Input: dimensioned drawing with shaded views. Units: mm. Origin: part minimum x, y, z. A direction names the side the tool comes from. Give positions to 0.01 mm unless a question says otherwise; leave off trailing zeros. Order: outer loops, then holes, each group sorted by start corner. A loop starts at its lowest first (then second) coordinate and runs counter-clockwise, first axis right, second up. Notation, with made-up numbers: (-30.5, 3.25) - (22.5, 3.25) arc R14 ccw to (22.5, 12.25) - close; hole circle Ø8 at (79.5, 72.5). An arc over 180 degrees is marked (long way). Use a Markdown table: item, result.
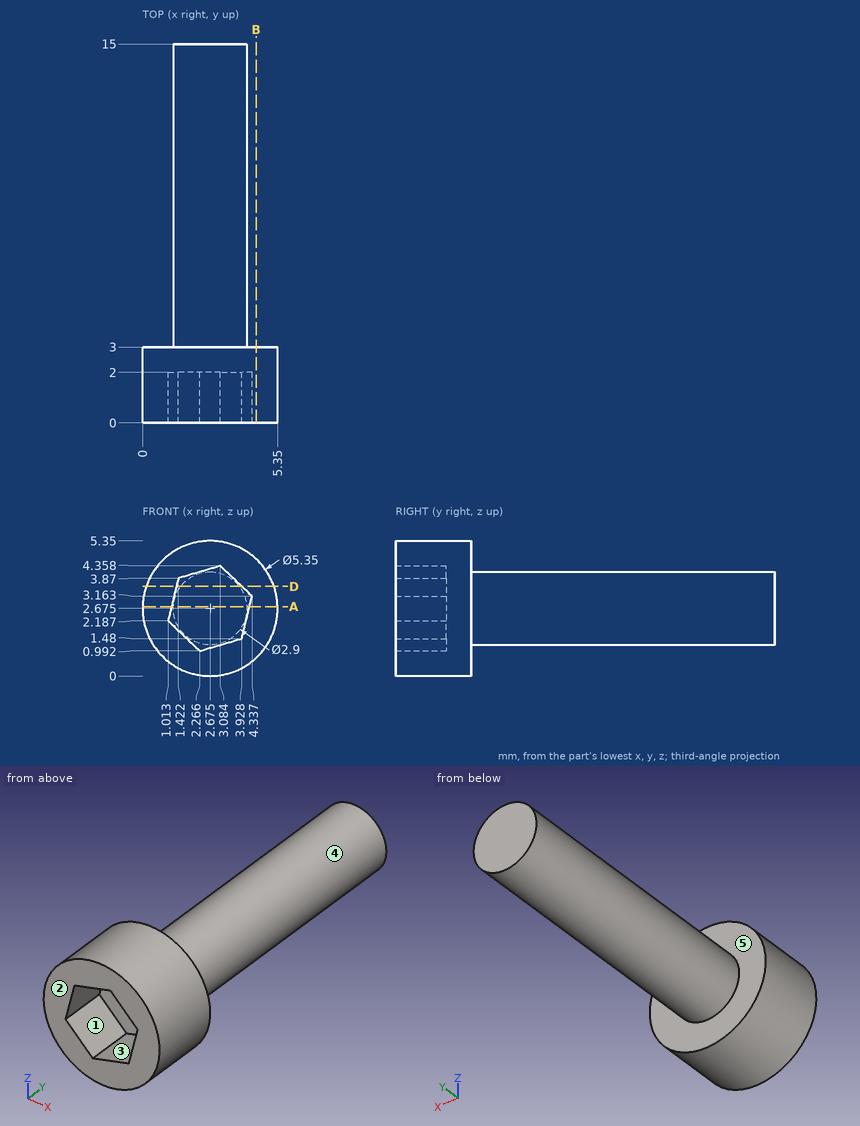
1. Section query A-A (z = 2.75). Return loops of the section in (x, y).
Response:
| item | result |
|---|---|
| outline | (0, 0) - (1.15, 0) - (1.15, 2) - (4.24, 2) - (4.24, 0) - (5.35, 0) - (5.35, 3) - (4.12, 3) - (4.12, 15) - (1.23, 15) - (1.23, 3) - (0, 3) - close |
2. Mould query, pull axis Z, two halves, no side actions, for the marked faces 3, 4 and 5. Classes: pulls with the +Z half, pulls with the -Z half, needs draft (parallel to the pull), parting line crosses it, or undercut.
Response:
| item | result |
|---|---|
| face 3 | undercut |
| face 4 | parting line crosses it |
| face 5 | needs draft |
3. Set-up query: the marked faces 1 and 2. Return all of +Z, -Z, +X, -X, +Y, -Y with unobstructed straight access to the full face (end or side cutting, diameter ignored); none if empty.
Response:
| item | result |
|---|---|
| face 1 | -Y |
| face 2 | +Z, -Z, +X, -X, -Y |
4. Material intervals for line 1 along Y through (x, z) = (4.05, 4.8); line 2 along Z through (x, y) = (1.5, 1) (1 decimal); line 3 along Z through (x, y) = (2.7, 7.75) (1 decimal), sorted ascending.
Response:
| item | result |
|---|---|
| line 1 | y = 0 to 3 |
| line 2 | z = 0.3 to 1.7, 3.9 to 5.1 |
| line 3 | z = 1.2 to 4.1 |
5. Section query D-D (z = 3.55). Return loops of the section in (x, y).
Response:
| item | result |
|---|---|
| outline | (0.15, 0) - (1.34, 0) - (1.34, 2) - (3.93, 2) - (3.93, 0) - (5.2, 0) - (5.2, 3) - (3.83, 3) - (3.83, 15) - (1.52, 15) - (1.52, 3) - (0.15, 3) - close |
6. Pin query (flat end, axial travel): pin 1 (1.7 mm diameter, centred on x = 3, z = 2.5, fed in from -Y); pin 2 (2 mm diameter, centred on y = 11.5, z = 3.5, fed in from +X) (3 decimals). Return the tip coordinate at first contact, or that it passes through.
Response:
| item | result |
|---|---|
| pin 1 | stops at y = 2 |
| pin 2 | stops at x = 4.125 |
7. Section query B-B (x = 4.5). Return loops of the section in (y, z), then the cut area to 3 significant figures.
Response:
| item | result |
|---|---|
| outline | (0, 0.72) - (3, 0.72) - (3, 4.63) - (0, 4.63) - close |
| area | 11.7 mm^2 |
